Autodesk Inventor part; units mm, degrees
ref_plane "YZ Plane" through (0, 0, 0) normal (1, 0, 0) x (0, 1, 0)
ref_plane "XZ Plane" through (0, 0, 0) normal (0, 1, 0) x (-1, 0, 0)
ref_plane "XY Plane" through (0, 0, 0) normal (0, 0, 1) x (1, 0, 0)
sketch "Sketch1" plane through (0, 0, 0) normal (0, 1, 0) x (-1, 0, 0)
  circle A0 centre (0, 0) radius 1.98
  dimension "d0" = 3.96
extrude "Extrusion1" add sketch "Sketch1" along normal blind 1.6
sketch "Sketch2" plane through (0, 1.6, 0) normal (0, 1, 0) x (1, 0, 0)
  line L0 (-0.35, -0.35) -> (-1.25, -0.35)
  line L1 (-1.25, -0.35) -> (-1.25, 0.35)
  line L2 (-1.25, 0.35) -> (-0.35, 0.35)
  line L3 (-0.35, 0.35) -> (-0.35, 1.25)
  line L4 (-0.35, 1.25) -> (0.35, 1.25)
  line L5 (0.35, 1.25) -> (0.35, 0.35)
  line L6 (0.35, 0.35) -> (1.25, 0.35)
  line L7 (1.25, 0.35) -> (1.25, -0.35)
  line L8 (1.25, -0.35) -> (0.35, -0.35)
  line L9 (0.35, -1.25) -> (-0.35, -1.25)
  line L10 (-0.35, -1.25) -> (-0.35, -0.35)
  line L11 (0.35, -0.35) -> (0.35, -1.25)
  point P0 (0, 0)
  point P1 (0, -1.25)
  point P2 (0, 1.25)
  point P3 (-1.25, 0)
  point P4 (1.25, 0)
  dimension "d3" = 2.5
  dimension "d4" = 2.5
  dimension "d5" = 1.25
  dimension "d6" = 1.25
  dimension "d7" = 0.7
  dimension "d8" = 0.7
extrude "Extrusion2" cut sketch "Sketch2" against normal blind 2
fillet "Fillet1" radius 1 1 edges at (1.98, 1.6, 0)
sketch "Sketch3" plane through (0, 0, 0) normal (0, -1, 0) x (1, 0, 0)
  circle A0 centre (0, 0) radius 1
  dimension "d12" = 2
extrude "Extrusion3" add sketch "Sketch3" along normal blind 10
thread "Thread1"
equation "\"d4\" = d3"
equation "\"d8\" = d7"
equation "\"d13\" = length"
equation "\"length\" = 10"
properties part number "M4_8mm" material "Stainless Steel"
Geometry: final body of the model. Coordinates: model frame, mm. A direction names the side the tool comes from. Coordinates: 2 decimals unless noted, no trailing zeros. Order: outer loops, then holes, each group sorted by start corner. A loop starts at its lowest first (then second) coordinate and runs counter-clockwise, first axis right, second up.
(1) Section query A-A (z = 0). State how many separate pieces and enclosed holes the cut face has, plus the area to 3 significant figures.
(2) Draft query along Z for faces 4 (the face through (0, -10, 0)), 5 (the face through (0, -5, 1)), 6 (the face through (0.35, 1, 1)), 7 (the face through (-1, 1, -0.35)). Return one class per face: pulls with the +Z half, pulls with the -Z half, needs draft (parallel to the pull), parting line crosses it, or undercut.
(3) Section query C-C (y = -1). Return the cut outline in (x, z), plus the area to 3 significant figures.
(4) Material intervals for probe 1 along Z at (x, y) = (0.55, 0.5); probe 2 along X at (y, z) = (0.5, -0.5); probe 3 along X at (y, z) = (-1.5, 0.9), sorted ascending.
(5) First-contact query: pin 1 (1 mm diameter, centred on x = 0.5, y = 1, fed in from +Z); pin 2 (1.5 mm diameter, centred on y = -6, z = 1.5, fed in from +X); pin 3 (1 mm diameter, centred on y = 1, z = 1, fed in from -X). Flat tips, straight axial feed; report the tip coordinate or a pass-through.
(6) Access query for faces 1 (the face through (0.429, 0.296, 1.933)), 2 (the face through (-1, 0, -1)), 3 (the face through (0.35, 1, -1)). Directions: +Z, -Z, +X, -X, +Y, -Y. A direction counts if a zero-diameter tool reaches every point of the face in a straight line with its end or side. Return the directions, or none.
Solution:
1. separate pieces: 3
1. enclosed holes: 0
1. area: 21.9 mm2
2. face 4: needs draft
2. face 5: parting line crosses it
2. face 6: undercut
2. face 7: undercut
3. outline: circle Ø2 at (0, 0)
3. area: 3.14 mm2
4. probe 1: z = -1.9 to -0.35, 0.35 to 1.9
4. probe 2: x = -1.92 to -0.35, 0.35 to 1.92
4. probe 3: x = -0.44 to 0.44
5. pin 1: stops at z = 1.97
5. pin 2: stops at x = 0.66
5. pin 3: stops at x = -1.89
6. face 1: +Y, -Y
6. face 2: -Y
6. face 3: +Y
